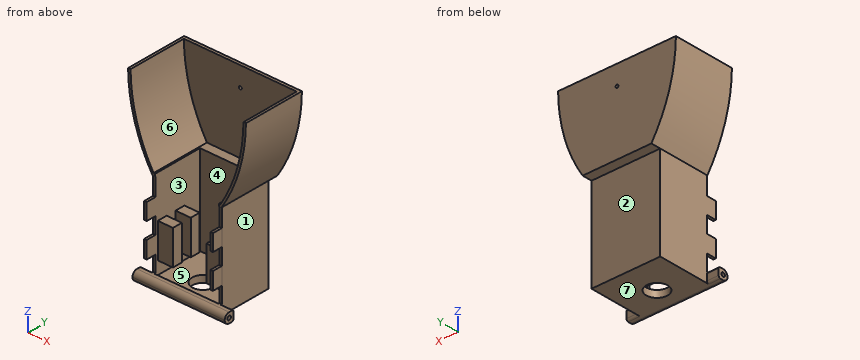
from build123d import *

# Parameters (mm, degrees)
SKETCH_1_W                = 70
SKETCH_1_H                = 70
EXTRUDE_1_DEPTH           = 180
SKETCH_3_W                = 65
SKETCH_3_H                = 65
CUT_EXTRUDE_1_DEPTH       = 173
SKETCH_4_R                = 10.95
CUT_EXTRUDE_2_DEPTH       = 137
SKETCH_5_W                = 50
SKETCH_5_H                = 55
CUT_EXTRUDE_3_DEPTH       = 137
SKETCH_6_W                = 35
SKETCH_6_H                = 10
EXTRUDE_2_DEPTH           = 18
CUT_EXTRUDE_4_DEPTH       = 200.321348581
CUT_EXTRUDE_4_DEPTH_BACK  = 200.321348581
SKETCH_7_W                = 70
SKETCH_7_H                = 20
SKETCH_9_W                = 70
SKETCH_9_H                = 180
EXTRUDE_3_DEPTH           = 2.5
EXTRUDE_4_DEPTH           = 10
EXTRUDE_4_DEPTH_BACK      = 53
CUT_EXTRUDE_7_DEPTH       = 60
SKETCH_18_W               = 65
SKETCH_18_H               = 47.5
CUT_EXTRUDE_12_DEPTH      = 105
CUT_EXTRUDE_13_DEPTH      = 105
CUT_EXTRUDE_13_DEPTH_BACK = 2.5
SKETCH_20_W               = 65
SKETCH_20_H               = 125.518576077
SKETCH_21_R               = 1.5
CUT_EXTRUDE_14_DEPTH      = 10
SKETCH_23_W               = 94
SKETCH_23_H               = 10
EXTRUDE_5_DEPTH           = 10
SKETCH_24_R               = 2
CUT_EXTRUDE_15_DEPTH      = 194
FILLET_1_R                = 2
FILLET_2_R                = 2
FILLET_3_R                = 2
FILLET_4_R                = 5
SKETCH_25_W               = 2.52996266
SKETCH_25_H               = 16.78546259
SKETCH_25_H_2             = 17.490734126
SKETCH_25_W_2             = 2.5
SKETCH_25_H_3             = 17.349679819
EXTRUDE_6_DEPTH           = 10


with BuildPart() as part:
    # 스케치1 → 보스-돌출1 (new body)
    with BuildSketch(Plane.XY):
        with Locations((35, -35)):
            Rectangle(SKETCH_1_W, SKETCH_1_H)
    extrude(amount=EXTRUDE_1_DEPTH)

    # 스케치3 → 컷-돌출1 (cut)
    with BuildSketch(Plane.XY.offset(180)):
        with Locations((35, -35)):
            Rectangle(SKETCH_3_W, SKETCH_3_H)
    extrude(amount=-CUT_EXTRUDE_1_DEPTH, mode=Mode.SUBTRACT)

    # 스케치4 → 컷-돌출2 (cut)
    with BuildSketch(Plane(origin=(0, 0, 0), x_dir=(-1, 0, 0), z_dir=(0, 0, -1))):
        with Locations((-35, -35)):
            Circle(SKETCH_4_R)
    extrude(amount=-CUT_EXTRUDE_2_DEPTH, mode=Mode.SUBTRACT)

    # 스케치5 → 컷-돌출3 (cut)
    with BuildSketch(Plane(origin=(70, 0, 0), x_dir=(0, 0, -1), z_dir=(1, 0, 0))):
        with Locations((-155, -35)):
            Rectangle(SKETCH_5_W, SKETCH_5_H)
    extrude(amount=-CUT_EXTRUDE_3_DEPTH, mode=Mode.SUBTRACT)

    # 스케치6 → 보스-돌출2 (add)
    with BuildSketch(Plane.ZY):
        with Locations((37.5, -25)):
            Rectangle(SKETCH_6_W, SKETCH_6_H)
        with Locations((37.5, -45)):
            Rectangle(SKETCH_6_W, SKETCH_6_H)
    extrude_2 = extrude(amount=-EXTRUDE_2_DEPTH)

    # 대칭 복사1: 보스-돌출2 across plane
    add(extrude_2.mirror(Plane(origin=(35, 0, 0), x_dir=(0, 0, 1), z_dir=(1, 0, 0))))

    # 스케치7 → 컷-돌출4 (cut, two sides: drawn at the far end of the back side and taken through both)
    with BuildSketch(Plane.XY.offset(7).offset(-CUT_EXTRUDE_4_DEPTH_BACK)):
        with Locations((35, -60)):
            Rectangle(SKETCH_7_W, SKETCH_7_H)
    extrude(amount=CUT_EXTRUDE_4_DEPTH + CUT_EXTRUDE_4_DEPTH_BACK, mode=Mode.SUBTRACT)

    # 스케치9 → 보스-돌출3 (add)
    with BuildSketch(Plane.XZ.offset(50)):
        with Locations((35, 90)):
            Rectangle(SKETCH_9_W, SKETCH_9_H)
    extrude(amount=EXTRUDE_3_DEPTH)

    # 스케치11 → 보스-돌출4 (add, two sides: drawn at the far end of the back side and taken through both)
    with BuildSketch(Plane(origin=(0, 0, 0), x_dir=(1, 0, 0), z_dir=(0, 1, 0)).offset(-EXTRUDE_4_DEPTH_BACK)):
        with BuildLine():
            Line((0, -95.320459485), (70, -95.320459485))
            ThreePointArc((70, -95.320459485), (88.456704779, -135.901627622), (95, -180))
            Line((95, -180), (-25, -180))
            ThreePointArc((-25, -180), (-18.456704779, -135.901627622), (0, -95.320459485))
        make_face()
    extrude(amount=EXTRUDE_4_DEPTH + EXTRUDE_4_DEPTH_BACK)

    # 스케치13 → 컷-돌출7 (cut)
    with BuildSketch(Plane.XZ.offset(53)):
        with BuildLine():
            Line((-22.5, 180), (92.5, 180))
            ThreePointArc((92.5, 180), (86.367270586, 137.316234441), (69.058371922, 97.820459485))
            Line((69.058371922, 97.820459485), (0.941628078, 97.820459485))
            ThreePointArc((0.941628078, 97.820459485), (-16.367270586, 137.316234441), (-22.5, 180))
        make_face()
    extrude(amount=-CUT_EXTRUDE_7_DEPTH, mode=Mode.SUBTRACT)

    # 스케치18 → 컷-돌출12 (cut)
    with BuildSketch(Plane(origin=(0, 0, 95.320459485), x_dir=(-1, 0, 0), z_dir=(0, 0, -1))):
        with Locations((-35, -26.25)):
            Rectangle(SKETCH_18_W, SKETCH_18_H)
    extrude(amount=-CUT_EXTRUDE_12_DEPTH, mode=Mode.SUBTRACT)

    # 스케치20 → 컷-돌출13 (cut, two sides: drawn at the far end of the back side and taken through both)
    with BuildSketch(Plane.XZ.offset(52.5).offset(-CUT_EXTRUDE_13_DEPTH_BACK)):
        with Locations((35, 69.759288039)):
            Rectangle(SKETCH_20_W, SKETCH_20_H)
    extrude(amount=CUT_EXTRUDE_13_DEPTH + CUT_EXTRUDE_13_DEPTH_BACK, mode=Mode.SUBTRACT)

    # 스케치21 → 컷-돌출14 (cut)
    with BuildSketch(Plane(origin=(0, 10, 0), x_dir=(1, 0, 0), z_dir=(0, 1, 0))):
        with Locations(Location((35, -160, 0), (0, 0, 270))):
            Circle(SKETCH_21_R)
    extrude(amount=-CUT_EXTRUDE_14_DEPTH, mode=Mode.SUBTRACT)

    # 스케치23 → 보스-돌출5 (add)
    with BuildSketch(Plane.XZ.offset(52.5)):
        with Locations((35, 5)):
            Rectangle(SKETCH_23_W, SKETCH_23_H)
    extrude(amount=EXTRUDE_5_DEPTH)

    # 스케치24 → 컷-돌출15 (cut)
    with BuildSketch(Plane.ZY.offset(12)):
        with Locations((4.937361109, -57.5)):
            Circle(SKETCH_24_R)
    extrude(amount=-CUT_EXTRUDE_15_DEPTH, mode=Mode.SUBTRACT)

    # 필렛1
    fillet_1_edges = [part.edges().sort_by_distance(p)[0] for p in [
        (35, -52.5, 10),
    ]]
    fillet(fillet_1_edges, radius=FILLET_1_R)

    # 필렛2
    fillet_2_edges = [part.edges().sort_by_distance(p)[0] for p in [
        (76, -52.5, 10),
        (-6, -52.5, 10),
    ]]
    fillet(fillet_2_edges, radius=FILLET_2_R)

    # 필렛3
    fillet_3_edges = [part.edges().sort_by_distance(p)[0] for p in [
        (-6, -52.5, 0),
        (76, -52.5, 0),
    ]]
    fillet(fillet_3_edges, radius=FILLET_3_R)

    # 필렛4
    fillet_4_edges = [part.edges().sort_by_distance(p)[0] for p in [
        (35, -62.5, 10),
        (35, -62.5, 0),
    ]]
    fillet(fillet_4_edges, radius=FILLET_4_R - 0.0001)  # a hair under: the kernel refuses the full size

    # 스케치25 → 보스-돌출6 (add)
    with BuildSketch(Plane.XZ.offset(52.5)):
        with Locations((68.76498133, 68.677635779)):
            Rectangle(SKETCH_25_W, SKETCH_25_H)
        with Locations((68.76498133, 34.895129139)):
            Rectangle(SKETCH_25_W, SKETCH_25_H_2)
        with Locations((1.25, 68.677635779)):
            Rectangle(SKETCH_25_W_2, SKETCH_25_H)
        with Locations((1.25, 34.965656293)):
            Rectangle(SKETCH_25_W_2, SKETCH_25_H_3)
    extrude(amount=EXTRUDE_6_DEPTH)


solid = part.part
Input: part model. Units: mm. Frame: model coordinates. Face numbers are marked on the shaded views. A direction names the side the tool comes from. Round coordinates to 2 decimals unless told otherwise and drop trailing zeros. Loops run counter-clockwise (first coordinate to the right, second up) from the corner with the lowest first, then second, coordinate; pieces in that order, holes last. Notation, with made-up numbers: M 41,49.5 L 92,49.5 A23 cw 92,65.5 Z; hole C 30.5,0 d6. An arc over 180 degrees is marked long. Answer as CSV lines item,"result". Start each with the question number.
(1) Line query: line 1 (Z direction, x = 17, y = -29); line 2 (Y direction, x = 35, z = 4.75); line 3 (X direction, y = -39.5, z = 60). Output: solid intervals per line, ascending. Write a range as [from, to].
(2) Reachability of the marked faces 4, 5, 6 and 7 from +Z, -Z, +X, -X, +Y, -Y: full face, straight path, thin tool, end or side. Return the list, or none.
(3) First-contact query: pin 1 (0.8 mm diameter, centred on x = 68, z = 20.5, fed in from -Y); pin 2 (24.5 mm diameter, centred on x = 55.5, z = 139, fed in from -Y); pin 3 (8 mm diameter, centred on x = 65, y = -42.5, fed in from +Z). Flat tips, straight axial feed; report the tip coordinate or a pass-through.
(4) Section A-A, the plane x = 73. State how many separate pieces and enclosed holes the cut face has, plus the area to 3 significant figures.
(5) Draft query along X for the marked faces 1, 2 and 3. Return one class per face: released by +X, released by -X, zero draft, split by the parting line, or undercut.
(6) Section C-C, the plane y = -10. Output: boundary loops of the cut face in (x, z).
Values found:
1,line 1,"z = [0, 7], [20, 55]"
1,line 2,"y = [-62.49, -59.49], [-55.51, -45.95], [-24.05, 0]"
1,line 3,"x = [0, 2.5], [67.5, 70]"
2,face 4,"+Z"
2,face 5,"none"
2,face 6,"+Z, -Y"
2,face 7,"-Z, +X, -X, +Y, -Y"
3,pin 1,"stops at y = -52.5"
3,pin 2,"stops at y = 7"
3,pin 3,"stops at z = 97.82"
4,separate pieces,"2"
4,enclosed holes,"1"
4,area,"579 mm²"
5,face 1,"released by +X"
5,face 2,"zero draft"
5,face 3,"undercut"
6,outline,"M -25,180 A160 ccw 0,95.32 L 0,0 L 70,0 L 70,95.32 A160 ccw 95,180 L 92.5,180 A160 cw 69.06,97.82 L 67.5,97.82 L 67.5,7 L 2.5,7 L 2.5,97.82 L 0.94,97.82 A160 cw -22.5,180 Z"
